Read the model definition and answer for the solid it produces. Units are mm, in the model's axes. A direction names the side the tool comes from. Give positions to 0.01 mm unless a question says otherwise; leave off trailing zeros. Order: outer loops, then holes, each group sorted by start corner. A loop starts at its lowest first (then second) coordinate and runs counter-clockwise, first axis right, second up. Notation, with made-up numbers: M 81.5,61.25 L 93.5,61.25 A25 cw 93.5,97.25 Z; hole C 16.25,89 d5. An arc over 180 degrees is marked long. One line per item, written item: value.
from build123d import *

# Parameters (mm, degrees)
BOSS_EXTRUDE1_DEPTH = 25
BOSS_EXTRUDE2_DEPTH = 25
SKETCH3_W           = 45
SKETCH3_H           = 35
BOSS_EXTRUDE3_DEPTH = 25


with BuildPart() as part:
    # Sketch1 → Boss-Extrude1 (new body)
    with BuildSketch(Plane(origin=(0, 0, 0), x_dir=(1, 0, 0), z_dir=(0, 1, 0))):
        Polygon((0, 0), (60, 0), (60, 35), (130, 35), (130, 80), (0, 80), align=None)
    extrude(amount=BOSS_EXTRUDE1_DEPTH)

    # Sketch2 → Boss-Extrude2 (add)
    with BuildSketch(Plane.ZY):
        Polygon((0, 40), (-35, 60), (-80, 60), (-80, 25), (0, 25), align=None)
    extrude(amount=-BOSS_EXTRUDE2_DEPTH)

    # Sketch3 → Boss-Extrude3 (add)
    with BuildSketch(Plane(origin=(130, 0, 0), x_dir=(0, 0, -1), z_dir=(1, 0, 0))):
        with Locations((57.5, 42.5)):
            Rectangle(SKETCH3_W, SKETCH3_H)
    extrude(amount=-BOSS_EXTRUDE3_DEPTH)


solid = part.part
1) Find section D-D, the plane x = 74.5. Write down the section's boundary in (y, z).
Reported:
outline: M 0,-80 L 25,-80 L 25,-35 L 0,-35 Z
2) Consider probe 1 along X at (y, z) = (52.5, -67.5); probe 2 along X at (y, z) = (35, -26.5). Determine where each line is inside the solid, lowest interval first.
Reported:
probe 1: x = 0 to 25, 105 to 130
probe 2: x = 0 to 25
3) Which of the six approach directions +Z, -Z, +X, -X, +Y, -Y give full straight-line access (tool end or side, diameter ignored) to faces 1 (the face through (105, 43, -57)), 2 (the face through (30, 15, 0)), 3 (the face through (60, 12, -17))?
Reported:
face 1: +Z, -Z, +Y
face 2: +Z, +X, -X, +Y, -Y
face 3: +Z, +X, +Y, -Y
4) Find section C-C, the plane y = 18. Write down the section's boundary in (x, z).
Reported:
outline: M 0,-80 L 130,-80 L 130,-35 L 60,-35 L 60,0 L 0,0 Z
5) Find section A-A, the plane y = 51.5. Write down the section's boundary in (x, z) (3 decimals), plus the area to 3 significant figures.
Reported:
outline: M 0,-80 L 25,-80 L 25,-20.125 L 0,-20.125 Z; M 105,-80 L 130,-80 L 130,-35 L 105,-35 Z
area: 2,620 mm^2
6) Each of these flat-tipped pins is pushed along its axis until it touches: pin 1 Ø10 at (x, y) = (106.5, 26) entering from +Z; pin 2 Ø7.5 at (y, z) = (10, -21) entering from +X; pin 3 Ø24 at (x, z) = (71.5, -37.5) entering from +Y. Where does it stop, or does it pass through?
Reported:
pin 1: stops at z = -35
pin 2: stops at x = 60
pin 3: stops at y = 25
7) Determine the mould class of faces 4 (the face through (66, 23, -80)), 5 (the face through (56, 25, -49)), 6 (the face through (130, 30, -57)) for opening direction X: +X half, -X half, draft (parallel to the pull), parting line (faces both ways), or undercut.
Reported:
face 4: draft
face 5: undercut
face 6: +X half
8) Find section B-B, the plane z = -68.5. Write down the section's boundary in (x, y).
Reported:
outline: M 0,0 L 130,0 L 130,60 L 105,60 L 105,25 L 25,25 L 25,60 L 0,60 Z
